from build123d import *

# Parameters (mm, degrees)
ESBO_O1_W                  = 500
ESBO_O1_H                  = 500
RESSALTO_EXTRUS_O1_DEPTH   = 10
CORTE_EXTRUS_O2_DEPTH      = 708.177488329
CORTE_EXTRUS_O2_DEPTH_BACK = 708.177488329
ESBO_O3_W                  = 25
ESBO_O3_H                  = 25
RESSALTO_EXTRUS_O2_DEPTH   = 100
ESBO_O4_W                  = 14
ESBO_O4_H                  = 14
RESSALTO_EXTRUS_O3_DEPTH   = 12
ESBO_O5_R                  = 7.24
RESSALTO_EXTRUS_O4_DEPTH   = 12
CHANFRO1_SIZE              = 1


with BuildPart() as part:
    # Esboço1 → Ressalto-extrusão1 (new body)
    with BuildSketch(Plane(origin=(0, 0, 0), x_dir=(1, 0, 0), z_dir=(0, 1, 0))):
        with Locations((250, 250)):
            Rectangle(ESBO_O1_W, ESBO_O1_H)
    extrude(amount=RESSALTO_EXTRUS_O1_DEPTH)

    # Esboço2 → Corte-extrusão2 (cut, two sides: drawn at the far end of the back side and taken through both)
    with BuildSketch(Plane(origin=(0, 10, 0), x_dir=(1, 0, 0), z_dir=(0, 1, 0)).offset(-CORTE_EXTRUS_O2_DEPTH_BACK)):
        with BuildLine():
            Line((232.85, 489.85), (232.85, 460.15))
            ThreePointArc((232.85, 460.15), (235, 458), (237.15, 460.15))
            Line((237.15, 460.15), (237.15, 489.85))
            ThreePointArc((237.15, 489.85), (235, 492), (232.85, 489.85))
        make_face()
        with BuildLine():
            Line((262.85, 489.85), (262.85, 460.15))
            ThreePointArc((262.85, 460.15), (265, 458), (267.15, 460.15))
            Line((267.15, 460.15), (267.15, 489.85))
            ThreePointArc((267.15, 489.85), (265, 492), (262.85, 489.85))
        make_face()
        with BuildLine():
            Line((489.85, 267.15), (460.15, 267.15))
            ThreePointArc((460.15, 267.15), (458, 265), (460.15, 262.85))
            Line((460.15, 262.85), (489.85, 262.85))
            ThreePointArc((489.85, 262.85), (492, 265), (489.85, 267.15))
        make_face()
        with BuildLine():
            Line((489.85, 237.15), (460.15, 237.15))
            ThreePointArc((460.15, 237.15), (458, 235), (460.15, 232.85))
            Line((460.15, 232.85), (489.85, 232.85))
            ThreePointArc((489.85, 232.85), (492, 235), (489.85, 237.15))
        make_face()
        with BuildLine():
            Line((267.15, 10.15), (267.15, 39.85))
            ThreePointArc((267.15, 39.85), (265, 42), (262.85, 39.85))
            Line((262.85, 39.85), (262.85, 10.15))
            ThreePointArc((262.85, 10.15), (265, 8), (267.15, 10.15))
        make_face()
        with BuildLine():
            Line((237.15, 10.15), (237.15, 39.85))
            ThreePointArc((237.15, 39.85), (235, 42), (232.85, 39.85))
            Line((232.85, 39.85), (232.85, 10.15))
            ThreePointArc((232.85, 10.15), (235, 8), (237.15, 10.15))
        make_face()
        with BuildLine():
            Line((10.15, 232.85), (39.85, 232.85))
            ThreePointArc((39.85, 232.85), (42, 235), (39.85, 237.15))
            Line((39.85, 237.15), (10.15, 237.15))
            ThreePointArc((10.15, 237.15), (8, 235), (10.15, 232.85))
        make_face()
        with BuildLine():
            Line((10.15, 262.85), (39.85, 262.85))
            ThreePointArc((39.85, 262.85), (42, 265), (39.85, 267.15))
            Line((39.85, 267.15), (10.15, 267.15))
            ThreePointArc((10.15, 267.15), (8, 265), (10.15, 262.85))
        make_face()
    extrude(amount=CORTE_EXTRUS_O2_DEPTH + CORTE_EXTRUS_O2_DEPTH_BACK, mode=Mode.SUBTRACT)

    # Esboço3 → Ressalto-extrusão2 (add)
    with BuildSketch(Plane(origin=(0, 10, 0), x_dir=(1, 0, 0), z_dir=(0, 1, 0))):
        with Locations((250, 250)):
            Rectangle(ESBO_O3_W, ESBO_O3_H)
    extrude(amount=RESSALTO_EXTRUS_O2_DEPTH)

    # Esboço4 → Ressalto-extrusão3 (add)
    with BuildSketch(Plane(origin=(0, 110, 0), x_dir=(1, 0, 0), z_dir=(0, 1, 0))):
        with Locations((250, 250)):
            Rectangle(ESBO_O4_W, ESBO_O4_H)
    extrude(amount=RESSALTO_EXTRUS_O3_DEPTH)

    # Esboço5 → Ressalto-extrusão4 (add)
    with BuildSketch(Plane(origin=(0, 122, 0), x_dir=(1, 0, 0), z_dir=(0, 1, 0))):
        with Locations((250, 250)):
            Circle(ESBO_O5_R)
    extrude(amount=-RESSALTO_EXTRUS_O4_DEPTH)

    # Chanfro1
    chanfro1_edges = [part.edges().sort_by_distance(p)[0] for p in [
        (243, 116, -257),
        (243, 116, -243),
        (257, 116, -243),
        (257, 116, -257),
    ]]
    chamfer(chanfro1_edges, length=CHANFRO1_SIZE)


solid = part.part
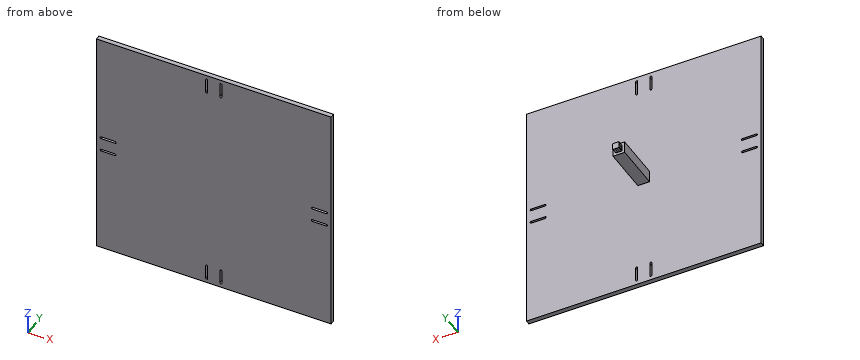
Can you work these out from the model? Positions are in its coordinate system, mm. Coordinates: 2 decimals unless noted, no trailing zeros. Loops run counter-clockwise (first coordinate to the right, second up) from the corner with the lowest first, then second, coordinate; pieces in that order, holes last. Notation, with made-up numbers: (75.5, -19) - (99.5, -19) arc R10 cw to (99.5, -11) - close; hole circle Ø9 at (74, 5). An arc over 180 degrees is marked (long way). Answer as a JSON object with one key per item and string values. Group by question number.
Item 1: If we section it at B-B (y = 17): List the corners of the cut face in (x, z) for me.
Item 2: For pin 1 (7.5 mm diameter, centred on x = 249.5, y = 41.5, fed in from -Z); pin 2 (3.5 mm diameter, centred on x = 246, y = 115, fed in from -Z); pin 3 (3.5 mm diameter, centred on y = 114, z = -254, fed in from +X), each with a flat end and sliding along its axis, tell me the tip position at first contact or that it passes through.
Item 3: If we section it at A-A (x = 138.5): List the corners of the cut face in (y, z) for me.
Item 4: If I drill on L1, parallel to Y at x = 201, z = -397; L2, parallel to Y at x = 262, z = -251.5; L3, parallel to X at y = 74.5, z = -241.5, over which ranges is the centre line in solid material (lowest first)? Write a range as from..to.
Returned:
{
 "1": {"outline": "(237.5, -262.5) - (262.5, -262.5) - (262.5, -237.5) - (237.5, -237.5) - close"},
 "2": {"pin 1": "stops at z = -262.5", "pin 2": "stops at z = -257", "pin 3": "stops at x = 257"},
 "3": {"outline": "(0, -500) - (10, -500) - (10, 0) - (0, 0) - close"},
 "4": {"L1": "y = 0..10", "L2": "y = 0..110", "L3": "x = 237.5..262.5"}
}
